Input: dimensioned drawing with shaded views. Units: mm. Origin: part minimum x, y, z. A direction names the side the tool comes from. Give positions to 0.01 mm unless a question says otherwise; leave off trailing zeros. Loops run counter-clockwise (first coordinate to the right, second up) from the corner with the lowest first, then second, coordinate; pieces in that order, holes last. Notation, with made-up numbers: M 72.25,6 L 116.25,6 A34 cw 116.25,41 Z; hole C 19.5,54.25 d6. An arc over 180 degrees is marked long. Use CSV: the item, a comma, the result in double quotes. Start each with the question number.
Q1. Section A-A, the plane y = 15. Output: boundary loops of the cut face in (x, z).
Q2. Pull-direction query (X, two-part tool) for the marked faces 1, 2, 3 and 4; classes: released by +X, released by -X, zero draft, split by the parting line, or undercut.
Q3. Section D-D, the plane z = 16.75. Output: boundary loops of the cut face in (x, y).
Q4. Pin query (flat end, axial travel): pin 1 (1.5 mm diameter, centred on y = 22, z = 6, fed in from -X); pin 2 (4 mm diameter, centred on x = 10, z = 13.5, fed in from +Y); pin 3 (5 mm diameter, centred on x = 5, z = 7.5, fed in from -Y). Return the tip coordinate at first contact, or that it passes through.
Q5. Reachability of the marked faces 5 and 6 from +Z, -Z, +X, -X, +Y, -Y: full face, straight path, thin tool, end or side. Return the list, or none.
Q6. Section C-C, the plane z = 13.5. Output: boundary loops of the cut face in (x, y).
Q7. Material intervals for line 1 along Y through (x, z) = (15, 8); line 2 along Y through (x, z) = (15, 16.5); line 3 along Z through (x, y) = (10.75, 21), sorted ascending.
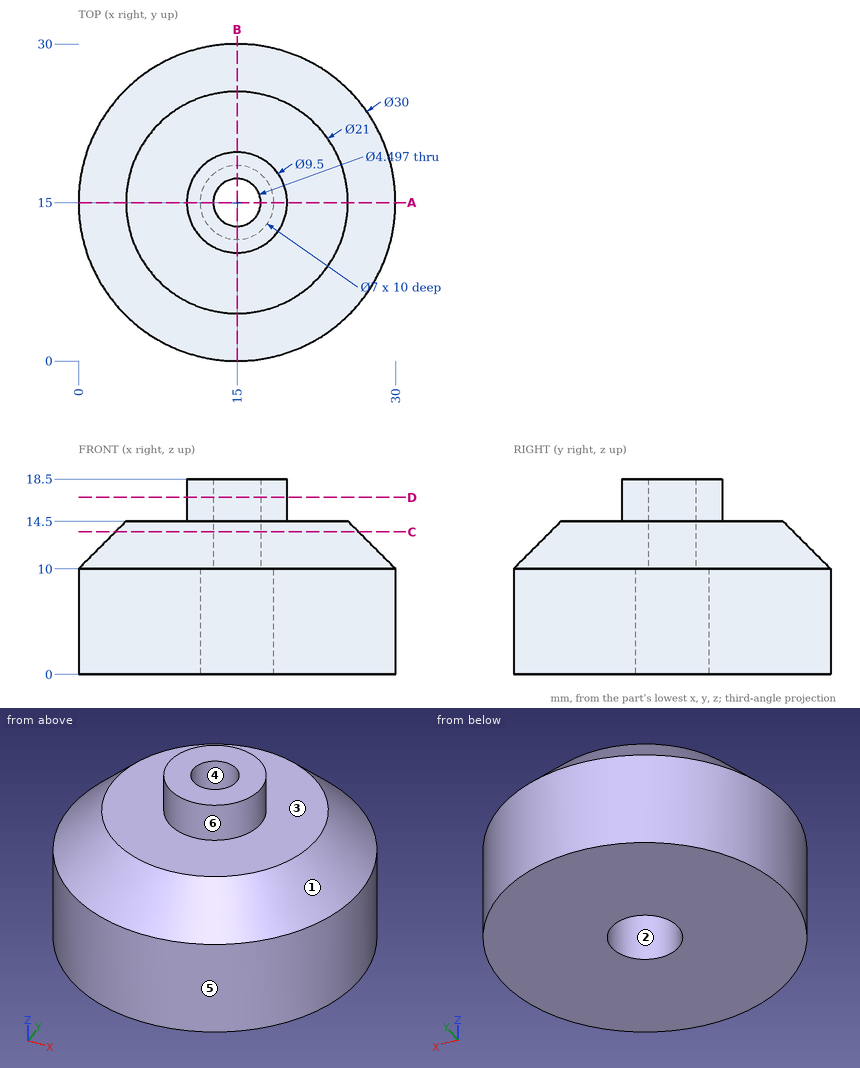
A:
1,outline,"M 0,0 L 11.5,0 L 11.5,10 L 12.75,10 L 12.75,18.5 L 10.25,18.5 L 10.25,14.5 L 4.5,14.5 L 0,10 Z; M 17.25,10 L 18.5,10 L 18.5,0 L 30,0 L 30,10 L 25.5,14.5 L 19.75,14.5 L 19.75,18.5 L 17.25,18.5 Z"
2,face 1,"split by the parting line"
2,face 2,"undercut"
2,face 3,"zero draft"
2,face 4,"undercut"
3,outline,"C 15,15 d9.5; hole C 15,15 d4.5"
4,pin 1,"x = 1.36"
4,pin 2,"y = 27.67"
4,pin 3,"y = 2.01"
5,face 5,"+Z, -Z"
5,face 6,"+Z"
6,outline,"C 15,15 d23; hole C 15,15 d4.5"
7,line 1,"0 to 11.5, 18.5 to 30"
7,line 2,"10.25 to 12.75, 17.25 to 19.75"
7,line 3,"0 to 14.5"
